```python
from build123d import *

# Parameters (mm, degrees)
SKETCH3_R           = 4
BOSS_EXTRUDE4_DEPTH = 3
SKETCH5_R           = 1.25
SKETCH5_R_2         = 5
CUT_EXTRUDE2_DEPTH  = 38.912717898
SKETCH6_R           = 1.75
CUT_EXTRUDE3_DEPTH  = 38.912717898
SKETCH8_R           = 2
CUT_EXTRUDE4_DEPTH  = 38.912717898


with BuildPart() as part:
    # Sketch3 → Boss-Extrude4 (new body)
    with BuildSketch(Plane.XY):
        with BuildLine():
            Line((-12.5, -15), (-12.5, 15))
            ThreePointArc((-12.5, 15), (-9.066038179, 23.290317201), (-0.775720978, 26.724279022))
            Line((-0.775720978, 26.724279022), (24.224279022, 26.724279022))
            ThreePointArc((24.224279022, 26.724279022), (26.717166406, 24.412726597), (24.600101889, 21.752689013))
            Line((24.600101889, 21.752689013), (19.656921871, 21.001043278))
            ThreePointArc((19.656921871, 21.001043278), (16.915054922, 19.634924783), (15.48452884, 16.926104149))
            Line((15.48452884, 16.926104149), (9.51547116, -16.926104149))
            ThreePointArc((9.51547116, -16.926104149), (-2.374739058, -26.049783342), (-12.5, -15))
        make_face()
        with Locations((-1.764648859, -19.076420455)):
            Circle(SKETCH3_R, mode=Mode.SUBTRACT)
    extrude(amount=BOSS_EXTRUDE4_DEPTH)

    # Sketch5 → Cut-Extrude2 (cut, through all)
    with BuildSketch(Plane.XY.offset(3)):
        with Locations((-9.5, 10)):
            Circle(SKETCH5_R)
        with Locations((9.5, 10)):
            Circle(SKETCH5_R)
        with Locations((0, 7)):
            Circle(SKETCH5_R_2)
    extrude(amount=-CUT_EXTRUDE2_DEPTH, mode=Mode.SUBTRACT)

    # Sketch6 → Cut-Extrude3 (cut, through all)
    with BuildSketch(Plane.XY.offset(3)):
        with Locations((24.224279022, 24.224279022)):
            Circle(SKETCH6_R)
    extrude(amount=-CUT_EXTRUDE3_DEPTH, mode=Mode.SUBTRACT)

    # Sketch8 → Cut-Extrude4 (cut, through all)
    with BuildSketch(Plane.XY.offset(3)):
        with Locations((11.295409365, 23.680851427)):
            Circle(SKETCH8_R)
        with Locations((-0.289384278, 25.919731906)):
            Circle(SKETCH8_R)
    extrude(amount=-CUT_EXTRUDE4_DEPTH, mode=Mode.SUBTRACT)


solid = part.part
```
Build history of the part. All positions in model axes, mm. Round coordinates to 2 decimals unless told otherwise and drop trailing zeros. Loops run counter-clockwise (first coordinate to the right, second up) from the corner with the lowest first, then second, coordinate; pieces in that order, holes last.
Item 1: Saw through at D-D (x = 3.5). List the corners of the cut face in (y, z).
Item 2: Saw through at A-A (x = -3). List the corners of the cut face in (y, z).
Item 3: Pin check, flat tips, straight feed: P1, Ø1.5, axis at x = -2.5, y = -9, coming from the -Z side; P2, Ø1, axis at x = 0, z = 1.5, coming from the -Y side. Stop position of each tip, or through.
Item 4: Saw through at B-B (y = 10). List the corners of the cut face in (x, z).
Item 5: Two-plate mould, pull along X, no slides. Class faces 1 (the face through (-2.63, -22.98, 1.48)), 2 (the face through (-2.145, -26.067, 1.479)), 3 (the face through (-9.619, 22.698, 1.479)): released by +X, released by -X, zero draft, split by the parting line, or undercut.
Item 6: Drill centre lines: line 1 along Y through (x, z) = (-2.5, 0.75); line 2 along X through (y, z) = (24.5, 1.45); line 3 along Y through (x, z) = (0, 1.15). Where is each one in solid material? Low to high.
Item 7: Saw through at C-C (z = 2). List the corners of the cut face in (x, y), then the cut area to 3 significant figures.
Worked answers:
1. outline: (-24.95, 0) - (3.43, 0) - (3.43, 3) - (-24.95, 3) - close; (10.57, 0) - (26.72, 0) - (26.72, 3) - (10.57, 3) - close
2. outline: (-25.98, 0) - (-22.88, 0) - (-22.88, 3) - (-25.98, 3) - close; (-15.27, 0) - (3, 0) - (3, 3) - (-15.27, 3) - close; (11, 0) - (26.51, 0) - (26.51, 3) - (11, 3) - close
3. P1: stops at z = 0
3. P2: stops at y = -26.05
4. outline: (-12.5, 0) - (-10.75, 0) - (-10.75, 3) - (-12.5, 3) - close; (-8.25, 0) - (-4, 0) - (-4, 3) - (-8.25, 3) - close; (4, 0) - (8.25, 0) - (8.25, 3) - (4, 3) - close; (10.75, 0) - (14.26, 0) - (14.26, 3) - (10.75, 3) - close
5. face 1: undercut
5. face 2: split by the parting line
5. face 3: released by -X
6. line 1: y = -26.04 to -23.01, -15.14 to 2.67, 11.33 to 26.6
6. line 2: x = -7.65 to -1.7, 1.12 to 9.47, 13.12 to 22.5, 25.95 to 26.71
6. line 3: y = -26 to -22.67, -15.49 to 2, 12 to 23.94
7. outline: (-12.5, -15) arc R11.09 ccw to (9.52, -16.93) - (15.48, 16.93) arc R5 cw to (19.66, 21) - (24.6, 21.75) arc R2.5 ccw to (24.22, 26.72) - (1.54, 26.72) arc R2 cw (long way) to (-2.15, 26.64) arc R11.72 ccw to (-12.5, 15) - close; hole circle Ø2.5 at (-9.5, 10); hole circle Ø8 at (-1.76, -19.08); hole circle Ø10 at (0, 7); hole circle Ø2.5 at (9.5, 10); hole circle Ø4 at (11.3, 23.68); hole circle Ø3.5 at (24.22, 24.22)
7. area: 1,130 mm2
